Part print with two shaded views. Sizes in mm from the minimum x, y, z corner. A direction names the side the tool comes from. Give positions to 0.01 mm unless a question says otherwise; leave off trailing zeros. Order: outer loops, then holes, each group sorted by start corner. A loop starts at its lowest first (then second) coordinate and runs counter-clockwise, first axis right, second up. Notation, with made-up numbers: M -12,21 L 13,21 A20 cw 13,49 Z; hole C 50,-2 d1. An arc over 180 degrees is marked long. Return JSON: item names as keys, results as strings.
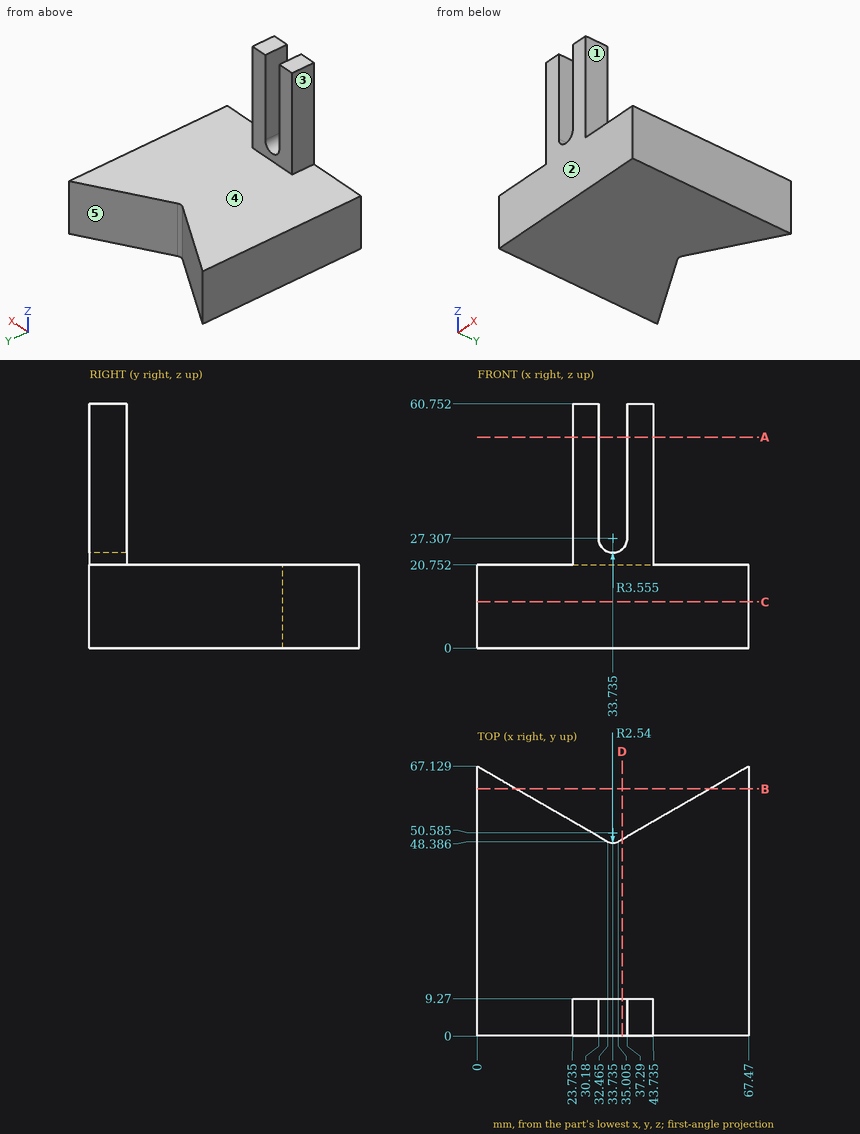
Q1. Two-plate mould, pull along X, no slides. Class the marked faces 3, 4 and 5: +X half, -X half, draft (parallel to the pull), parting line (faces both ways), or undercut.
Established:
{"face 3": "-X half", "face 4": "draft", "face 5": "undercut"}
Q2. Band-saw the part on C-C (z = 11.5). Give the cut face in (x, y) (1 decimal).
Established:
{"outline": "M 0,0 L 67.5,0 L 67.5,67.1 L 35,48.4 A2.5 cw 32.5,48.4 L 0,67.1 Z"}
Q3. Pin check, flat tips, straight feed: pin 1 (6 mm diameter, centred on y = 32.5, z = 18, fed in from -X); pin 2 (6 mm diameter, centred on x = 37.5, z = 48.5, fed in from +Y); pin 3 (3 mm diameter, centred on y = 6, z = 46.5, fed in from -X) (3 decimals); pin 4 (5 mm diameter, centred on x = 34, y = 25.5, fed in from +Z). Stop position of each tip, or through.
Established:
{"pin 1": "stops at x = 0", "pin 2": "stops at y = 9.27", "pin 3": "stops at x = 23.735", "pin 4": "stops at z = 20.75"}
Q4. Band-saw the part on D-D (x = 36). Give the cut face in (y, z), then the cut area to 3 significant figures.
Established:
{"outline": "M 0,0 L 48.96,0 L 48.96,20.75 L 9.27,20.75 L 9.27,24.57 L 0,24.57 Z", "area": "1,050 mm²"}
Q5. Band-saw the part on B-B (y = 61.5). Give the cut face in (x, z), then the cut area to 3 significant figures.
Established:
{"outline": "M 0,0 L 9.75,0 L 9.75,20.75 L 0,20.75 Z; M 57.72,0 L 67.47,0 L 67.47,20.75 L 57.72,20.75 Z", "area": "405 mm²"}
Q6. Band-saw the part on A-A (z = 52.5). Give the cut face in (x, y) (1 decimal).
Established:
{"outline": "M 23.7,0 L 30.2,0 L 30.2,9.3 L 23.7,9.3 Z; M 37.3,0 L 43.7,0 L 43.7,9.3 L 37.3,9.3 Z"}
Q7. Probe line 1 along Z through (x, y) = (57.5, 49); line 2 along X through (y, z) = (3.5, 25.5) (1 decimal); line 3 along X through (y, z) = (50, 17.5). List the from-to ranges inside material, lowest first.
Established:
{"line 1": "z = 0 to 20.75", "line 2": "x = 23.7 to 30.7, 36.8 to 43.7", "line 3": "x = 0 to 29.67, 37.8 to 67.47"}
Q8. 3-axis set-ups, long thin cutter, end or side, ignore diameter. For the marked faces 1 and 2: which of +Z, -Z, +X, -X, +Y, -Y reach the whole face in a straight line?
Established:
{"face 1": "+Z, +X, +Y, -Y", "face 2": "+Z, -Z, +X, -X, -Y"}
